Here's the drawing with two shaded views (mm, measured from the low corner). I have some questions. A direction names the side the tool comes from. Give positions to 0.01 mm unless a question says otherwise; leave off trailing zeros. Loops run counter-clockwise (first coordinate to the right, second up) from the corner with the lowest first, then second, coordinate; pieces in that order, holes last. Notation, with made-up numbers: M 45.5,77.25 L 57.5,77.25 A28 cw 57.5,110.25 Z; hole C 9.5,38 d7. An arc over 180 degrees is marked long. Put each result on its own line as item: value. Start each with the question number.
1) For P1, Ø7.5, axis at x = 111, z = 68, coming from the -Y side, with a flat end and sliding along its axis, tell me the tip position at first contact or that it passes through.
2) Imagine slicing it at D-D (z = 41). Write out the boundary of the cut face in (x, y), then the cut area to 3 significant figures.
3) Imagine slicing it at B-B (x = 30.5). Write out the boundary of the cut face in (y, z).
4) Imagine slicing it at C-C (z = 71). Write out the boundary of the cut face in (x, y), then the cut area to 3 significant figures.
5) Imagine slicing it at A-A (y = 98). Write out the boundary of the cut face in (x, z).
6) Please list where these lines run through material, in increasing order: line 1 along X through (y, z) = (92, 57.5); line 2 along Z through (x, y) = (45, 18); line 3 along Y through (x, z) = (132, 7.5). Write a range as from..to.
7) For the marked faces 1, 2 and 3, which set-ups out of +Z, -Z, +X, -X, +Y, -Y let a thin tool reach every point of the face, with its end or its side?
8) If we mould it in two halves opening along X, with no side actions, what happens to the marked faces 4, 5 and 6? For each: +X half, -X half, draft (parallel to the pull), parting line (faces both ways), or undercut.
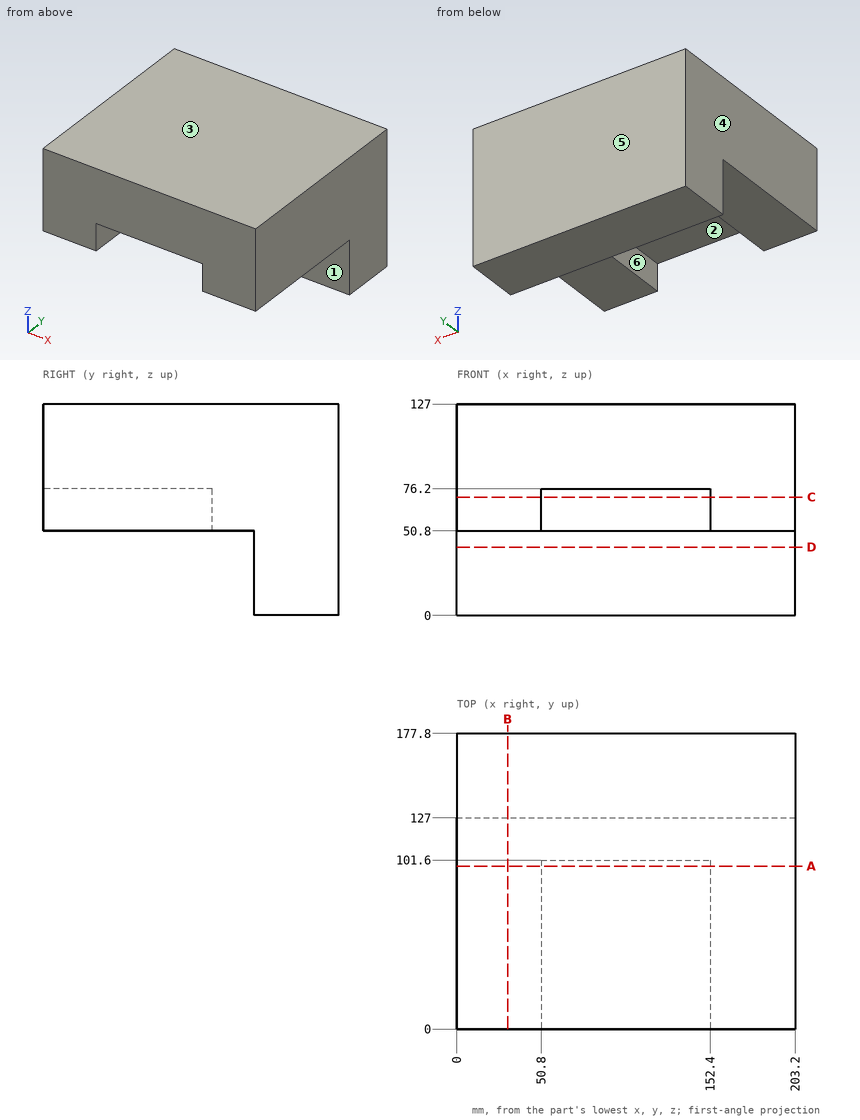
Recorded:
1. P1: y = 101.6
2. outline: M 0,127 L 203.2,127 L 203.2,177.8 L 0,177.8 Z
2. area: 10,300 mm²
3. outline: M 0,50.8 L 127,50.8 L 127,0 L 177.8,0 L 177.8,127 L 0,127 Z
4. outline: M 0,0 L 50.8,0 L 50.8,101.6 L 152.4,101.6 L 152.4,0 L 203.2,0 L 203.2,177.8 L 0,177.8 Z
4. area: 25,800 mm²
5. outline: M 0,50.8 L 50.8,50.8 L 50.8,76.2 L 152.4,76.2 L 152.4,50.8 L 203.2,50.8 L 203.2,127 L 0,127 Z
6. line 1: 0..50.8, 152.4..203.2
6. line 2: 50.8..127
6. line 3: 127..177.8
7. face 1: -Z, +X, -X, -Y
7. face 2: -Z, -Y
7. face 3: +Z, +X, -X, +Y, -Y
8. face 4: -X half
8. face 5: draft
8. face 6: undercut
